Can you work these out from the model? Positions are in its coordinate system, mm. Face numbers are marked on the shaded views. A direction names the side the tool comes from. Give positions to 0.01 mm unless a question says otherwise; leave off trailing zeros. Order: outer loops, then holes, each group sorted by start corner. A loop starts at its lowest first (then second) coordinate and runs counter-clockwise, first axis right, second up. Notation, with made-up numbers: (72, 15) - (107, 15) arc R20 cw to (107, 29) - close; hole circle Ø10 at (-32.75, 48). An arc over 180 degrees is marked (long way). Return JSON: item names as keys, results as strings.
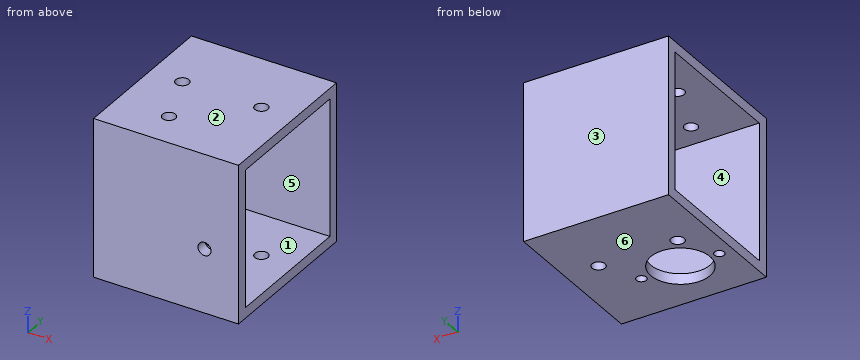
```python
from build123d import *

# Parameters (mm, degrees)
BOSS_EXTRUDE1_DEPTH      = 3.81
BOSS_EXTRUDE1_DEPTH_BACK = 1.27
SKETCH1_R                = 14.2748
SKETCH1_R_2              = 2.3876
SKETCH1_R_3              = 3.175
SKETCH2_W                = 69.85
SKETCH2_H                = 5.08
BOSS_EXTRUDE2_DEPTH      = 66.04
SKETCH3_W                = 69.85
SKETCH3_H                = 5.588
BOSS_EXTRUDE3_DEPTH      = 66.04
SKETCH4_W                = 69.85
SKETCH4_H                = 76.2
SKETCH4_R                = 3.175
BOSS_EXTRUDE4_DEPTH      = 5.08
CUT_EXTRUDE1_REACH       = 117.744
SKETCH6_R                = 3.174999999
SKETCH8_R                = 3.175
CUT_EXTRUDE2_DEPTH       = 102.545692986


with BuildPart() as part:
    # Sketch1 → Boss-Extrude1 (new, two sides: drawn at the far end of the back side and taken through both)
    with BuildSketch(Plane.XY.offset(-BOSS_EXTRUDE1_DEPTH_BACK)):
        Polygon((-25.4, 43.942), (-25.4, 50.292), (44.45, 50.292), (44.45, 24.892), (44.45, -25.908), (-25.4, -25.908), align=None)
        Circle(SKETCH1_R, mode=Mode.SUBTRACT)
        with Locations((18.7833, 0)):
            Circle(SKETCH1_R_2, mode=Mode.SUBTRACT)
        with Locations((-18.7833, 0)):
            Circle(SKETCH1_R_2, mode=Mode.SUBTRACT)
        with Locations((28.430863033, 17.78)):
            Circle(SKETCH1_R_3, mode=Mode.SUBTRACT)
    extrude(amount=BOSS_EXTRUDE1_DEPTH + BOSS_EXTRUDE1_DEPTH_BACK)

    # Sketch2 → Boss-Extrude2 (add)
    with BuildSketch(Plane.XY.offset(3.81)):
        with Locations((9.525, 47.752)):
            Rectangle(SKETCH2_W, SKETCH2_H)
    extrude(amount=BOSS_EXTRUDE2_DEPTH)

    # Sketch3 → Boss-Extrude3 (add)
    with BuildSketch(Plane.XY.offset(3.81)):
        with Locations((9.525, -23.114)):
            Rectangle(SKETCH3_W, SKETCH3_H)
    extrude(amount=BOSS_EXTRUDE3_DEPTH)

    # Sketch4 → Boss-Extrude4 (add)
    with BuildSketch(Plane.XY.offset(69.85)):
        with Locations((9.525, 12.192)):
            Rectangle(SKETCH4_W, SKETCH4_H)
        with Locations((28.430863033, 17.78)):
            Circle(SKETCH4_R, mode=Mode.SUBTRACT)
        with Locations((0, -8.2296)):
            Circle(SKETCH4_R, mode=Mode.SUBTRACT)
    extrude(amount=BOSS_EXTRUDE4_DEPTH)

    # Sketch6 → Cut-Extrude1 (cut, up to next)
    with BuildSketch(Plane.XZ.offset(25.908), mode=Mode.PRIVATE) as cut_extrude1_sk1:
        with Locations(Location((28.068770575, 29.478784222, 0), (0, 0, 270))):
            Circle(SKETCH6_R)
    cut_extrude1_tool1 = extrude(cut_extrude1_sk1.sketch, amount=-CUT_EXTRUDE1_REACH, mode=Mode.PRIVATE) & part.part
    add(cut_extrude1_tool1.solids().sort_by_distance((28.068771, -25.908, 29.478784))[0], mode=Mode.SUBTRACT)

    # Sketch8 → Cut-Extrude2 (cut, through all)
    with BuildSketch(Plane.XY.offset(74.93)):
        with Locations((-9.669136967, 17.78)):
            Circle(SKETCH8_R)
    extrude(amount=-CUT_EXTRUDE2_DEPTH, mode=Mode.SUBTRACT)


solid = part.part
```
1. Suppose I cut it at D-D (x = 35). List the corners of the cut face in (y, z) for me.
Checks:
{"outline": "(-25.91, -1.27) - (50.29, -1.27) - (50.29, 74.93) - (-25.91, 74.93) - close; hole (-20.32, 3.81) - (45.21, 3.81) - (45.21, 69.85) - (-20.32, 69.85) - close"}
2. For pin 1 Ø8.5 at (x, y) = (0, -8.23) entering from -Z; pin 2 Ø4 at (x, y) = (-9.67, 17.78) entering from -Z; pin 3 Ø4 at (x, z) = (28.07, 29.48) entering from -Y, each with a flat end and sliding along its axis, tell me the tip position at first contact or that it passes through.
Checks:
{"pin 1": "z = 69.85", "pin 2": "through", "pin 3": "y = 45.21"}
3. Suppose I cut it at B-B (y = 17.78). List the corners of the cut face in (x, z) for me, plus the area to 3 significant figures.
Checks:
{"outline": "(-25.4, -1.27) - (-12.84, -1.27) - (-12.84, 3.81) - (-25.4, 3.81) - close; (-25.4, 69.85) - (-12.84, 69.85) - (-12.84, 74.93) - (-25.4, 74.93) - close; (-6.49, -1.27) - (25.26, -1.27) - (25.26, 3.81) - (-6.49, 3.81) - close; (-6.49, 69.85) - (25.26, 69.85) - (25.26, 74.93) - (-6.49, 74.93) - close; (31.61, -1.27) - (44.45, -1.27) - (44.45, 3.81) - (31.61, 3.81) - close; (31.61, 69.85) - (44.45, 69.85) - (44.45, 74.93) - (31.61, 74.93) - close", "area": "581 mm^2"}
4. On a 3-axis mill with a long thin cutter (end or side, diameter ignored), from which of +Z, -Z, +X, -X, +Y, -Y can I reach the whole of each face in a straight line? I mean the marked faces 5 and 6. Say none if no direction works.
Checks:
{"face 5": "+X, -X", "face 6": "-Z, +X, -X, +Y, -Y"}
5. Thinking about a two-plate mould opening in Y: for the marked faces 1, 2, 3 and 4, which applies, +Y half, -Y half, draft (parallel to the pull), parting line (faces both ways), or undercut?
Checks:
{"face 1": "undercut", "face 2": "draft", "face 3": "+Y half", "face 4": "undercut"}
6. If I drill on L1, parallel to Y at x = -1, z = 41; L2, parallel to Z at x = 19.5, y = 18, over which ranges is the centre line in solid material (lowest first)? Write a range as [from, to].
Checks:
{"L1": "[-25.91, -20.32], [45.21, 50.29]", "L2": "[-1.27, 3.81], [69.85, 74.93]"}
7. Suppose I cut it at A-A (z = 20). List the corners of the cut face in (x, y) for me.
Checks:
{"outline": "(-25.4, -25.91) - (44.45, -25.91) - (44.45, -20.32) - (-25.4, -20.32) - close; (-25.4, 45.21) - (44.45, 45.21) - (44.45, 50.29) - (-25.4, 50.29) - close"}
8. Suppose I cut it at C-C (x = 0). List the corners of the cut face in (y, z) for me.
Checks:
{"outline": "(-25.91, -1.27) - (-14.27, -1.27) - (-14.27, 3.81) - (-20.32, 3.81) - (-20.32, 69.85) - (-11.4, 69.85) - (-11.4, 74.93) - (-25.91, 74.93) - close; (-5.05, 69.85) - (45.21, 69.85) - (45.21, 3.81) - (14.27, 3.81) - (14.27, -1.27) - (50.29, -1.27) - (50.29, 74.93) - (-5.05, 74.93) - close"}
